Source: CAD feature listing. Evaluate the final solid. Frame: model axes, mm. A direction names the side the tool comes from. Round coordinates to 2 decimals unless told otherwise and drop trailing zeros. Write each loop counter-clockwise with the first axis right and the second up, starting at its lowest first coordinate (ties: lowest second). Pieces come first, ordered by that corner, then holes. Notation, with made-up numbers: M -26.75,-30 L 6.25,-30 A4 cw 6.25,-24 Z; hole C -11.5,60.5 d10. An arc over 180 degrees is marked long. Answer in a Markdown table with one row per item. Add a question column.
Item 1: Cut plane A-A on z = 0. Return loops of the section in (x, y), and give its area (4 significant figures).
Item 2: Set-up query: faces 1 (the face through (6, 1, 2)), 2 (the face through (8.63, 0.49, -2.72)). Return all of +Z, -Z, +X, -X, +Y, -Y with unobstructed straight access to the full face (end or side cutting, diameter ignored); none if empty.
Item 3: Cut plane D-D on z = 4.75. Return loops of the section in (x, y).
Item 4: Material intervals for probe 1 along Y at (x, z) = (-2.5, 6.5); probe 2 along X at (y, z) = (1.15, 0), sorted ascending.
Item 5: Contact query for flat-ended pins moving along their axis: pin 1 (4.5 mm diameter, centred on x = 0, z = 0, fed in from +Y); pin 2 (1 mm diameter, centred on x = 0.5, y = 3.5, fed in from -Z); pin 3 (2 mm diameter, centred on y = 3.5, z = -6.5, fed in from -X); pin 4 (3 mm diameter, centred on y = 5.5, z = 4.5, fed in from +X). Output: stop coordinate, or through.
Item 6: Cut plane C-C on y = 2.75. Return loops of the section in (x, z), and give its area (3 significant figures).
Item 7: Cut plane B-B on x = 0. Return loops of the section in (y, z).
from build123d import *

# Parameters (mm, degrees)
SKETCH1_R           = 9.05
SKETCH1_R_2         = 6.05
SKETCH1_R_3         = 2.5
BOSS_EXTRUDE1_DEPTH = 1
BOSS_EXTRUDE2_START = 1
SKETCH1_3_R         = 6.05
SKETCH1_3_R_2       = 2.5
BOSS_EXTRUDE2_DEPTH = 3.25


with BuildPart() as part:
    # Sketch1 → Boss-Extrude1 (new body)
    with BuildSketch(Plane(origin=(0, 0, 0), x_dir=(1, 0, 0), z_dir=(0, 1, 0))):
        Circle(SKETCH1_R)
        Circle(SKETCH1_R_2, mode=Mode.SUBTRACT)
        Circle(SKETCH1_R_2)
        Circle(SKETCH1_R_3, mode=Mode.SUBTRACT)
    extrude(amount=BOSS_EXTRUDE1_DEPTH)

    # Sketch1<3> → Boss-Extrude2 (add)
    with BuildSketch(Plane(origin=(0, 0, 0), x_dir=(1, 0, 0), z_dir=(0, 1, 0)).offset(BOSS_EXTRUDE2_START)):
        Circle(SKETCH1_3_R)
        Circle(SKETCH1_3_R_2, mode=Mode.SUBTRACT)
    extrude(amount=BOSS_EXTRUDE2_DEPTH)

    # Mirror2: part across plane


with BuildPart() as part_1:
    add(part.part)
    add(part.part.mirror(Plane.ZX.offset(4.25)))


solid = part_1.part
Results below:
| question | item | result |
|---|---|---|
| 1 | outline | M -9.05,0 L -2.5,0 L -2.5,8.5 L -9.05,8.5 L -9.05,7.5 L -6.05,7.5 L -6.05,1 L -9.05,1 Z; M 2.5,0 L 9.05,0 L 9.05,1 L 6.05,1 L 6.05,7.5 L 9.05,7.5 L 9.05,8.5 L 2.5,8.5 Z |
| 1 | area | 72.35 mm2 |
| 2 | face 1 | none |
| 2 | face 2 | +Y, -Y |
| 3 | outline | M -7.7,0 L 7.7,0 L 7.7,1 L 3.75,1 L 3.75,7.5 L 7.7,7.5 L 7.7,8.5 L -7.7,8.5 L -7.7,7.5 L -3.75,7.5 L -3.75,1 L -7.7,1 Z |
| 4 | probe 1 | 0 to 1, 7.5 to 8.5 |
| 4 | probe 2 | -6.05 to -2.5, 2.5 to 6.05 |
| 5 | pin 1 | through |
| 5 | pin 2 | z = -6.05 |
| 5 | pin 3 | x = -2.52 |
| 5 | pin 4 | x = 5.25 |
| 6 | outline | C 0,0 d12.1; hole C 0,0 d5 |
| 6 | area | 95.4 mm2 |
| 7 | outline | M 0,-9.05 L 1,-9.05 L 1,-6.05 L 7.5,-6.05 L 7.5,-9.05 L 8.5,-9.05 L 8.5,-2.5 L 0,-2.5 Z; M 0,2.5 L 8.5,2.5 L 8.5,9.05 L 7.5,9.05 L 7.5,6.05 L 1,6.05 L 1,9.05 L 0,9.05 Z |
